```python
from build123d import *

# Parameters (mm, degrees)
CYLINDER893_R           = 1.6
CYLINDER893_DEPTH       = 10
CYLINDER893_PITCH_ANGLE = 90
CYLINDER894_R           = 1.6
CYLINDER894_DEPTH       = 10
CYLINDER894_PITCH_ANGLE = 90
CYLINDER896_R           = 3.1
CYLINDER896_DEPTH       = 2.5
CYLINDER896_PITCH_ANGLE = 90
CYLINDER895_R           = 3.1
CYLINDER895_DEPTH       = 2.5
CYLINDER895_PITCH_ANGLE = 90
BOX550_W                = 41
BOX550_H                = 41
BOX550_DEPTH            = 21
CYLINDER891_R           = 6
CYLINDER891_DEPTH       = 11
CYLINDER891_ROLL_ANGLE  = 90
CYLINDER945_R           = 7
CYLINDER945_DEPTH       = 5
CYLINDER945_ROLL_ANGLE  = 90
BOX559_W                = 10
BOX559_H                = 10
BOX559_DEPTH            = 17
CYLINDER693_R           = 1.2
CYLINDER693_DEPTH       = 10
CYLINDER693_ROLL_ANGLE  = 90
CYLINDER692_R           = 1.2
CYLINDER692_DEPTH       = 10
CYLINDER692_ROLL_ANGLE  = 90
CYLINDER697_R           = 1.25
CYLINDER697_DEPTH       = 15
CYLINDER697_PITCH_ANGLE = 90
CYLINDER695_R           = 1.25
CYLINDER695_DEPTH       = 11
CYLINDER695_PITCH_ANGLE = 90
CYLINDER696_R           = 1.25
CYLINDER696_DEPTH       = 15
CYLINDER696_PITCH_ANGLE = 90
CYLINDER694_R           = 1.25
CYLINDER694_DEPTH       = 11
CYLINDER694_PITCH_ANGLE = 90
BOX472_W                = 16
BOX472_H                = 60
BOX472_DEPTH            = 17
FILLET333_R             = 3
BOX473_W                = 10
BOX473_H                = 63
BOX473_DEPTH            = 25.5
FILLET332_R             = 3


with BuildPart() as cylinder1049:
    # Cylinder893 → Cylinder893 (new body)
    with BuildSketch(Plane.XY):
        Circle(CYLINDER893_R)
    extrude(amount=CYLINDER893_DEPTH)


with BuildPart() as cylinder1049_1:
    # Cylinder893 pitch: moved
    add(cylinder1049.part.rotate(Axis((0, 0, 0), (0, 1, 0)), CYLINDER893_PITCH_ANGLE))


with BuildPart() as cylinder1049_2:
    # Cylinder893 placement: moved
    add(cylinder1049_1.part.moved(Location((13.5, 83, -11))))


with BuildPart() as cylinder1050:
    # Cylinder894 → Cylinder894 (new body)
    with BuildSketch(Plane.XY):
        Circle(CYLINDER894_R)
    extrude(amount=CYLINDER894_DEPTH)


with BuildPart() as cylinder1050_1:
    # Cylinder894 pitch: moved
    add(cylinder1050.part.rotate(Axis((0, 0, 0), (0, 1, 0)), CYLINDER894_PITCH_ANGLE))


with BuildPart() as cylinder1050_2:
    # Cylinder894 placement: moved
    add(cylinder1050_1.part.moved(Location((13.5, 91, -11))))


with BuildPart() as cylinder1052:
    # Cylinder896 → Cylinder896 (new body)
    with BuildSketch(Plane.XY):
        Circle(CYLINDER896_R)
    extrude(amount=CYLINDER896_DEPTH)


with BuildPart() as cylinder1052_1:
    # Cylinder896 pitch: moved
    add(cylinder1052.part.rotate(Axis((0, 0, 0), (0, 1, 0)), CYLINDER896_PITCH_ANGLE))


with BuildPart() as cylinder1052_2:
    # Cylinder896 placement: moved
    add(cylinder1052_1.part.moved(Location((13.5, 83, -11))))


with BuildPart() as fusion593:
    # Cylinder895 → Cylinder895 (new body)
    with BuildSketch(Plane.XY):
        Circle(CYLINDER895_R)
    extrude(amount=CYLINDER895_DEPTH)


with BuildPart() as fusion593_1:
    # Cylinder895 pitch: moved
    add(fusion593.part.rotate(Axis((0, 0, 0), (0, 1, 0)), CYLINDER895_PITCH_ANGLE))


with BuildPart() as fusion593_2:
    # Cylinder895 placement: moved
    add(fusion593_1.part.moved(Location((13.5, 91, -11))))

    # Fusion593: union Cylinder1049, Cylinder1050, Cylinder1052
    add(cylinder1049_2.part)
    add(cylinder1050_2.part)
    add(cylinder1052_2.part)


with BuildPart() as cube741:
    # Box550 → Box550 (new body)
    with BuildSketch(Plane(origin=(19.5, 64.5, -21.5), x_dir=(1, 0, 0), z_dir=(0, 0, 1))):
        with Locations((20.5, 20.5)):
            Rectangle(BOX550_W, BOX550_H)
    extrude(amount=BOX550_DEPTH)


with BuildPart() as cylinder1048:
    # Cylinder891 → Cylinder891 (new body)
    with BuildSketch(Plane.XY):
        Circle(CYLINDER891_R)
    extrude(amount=CYLINDER891_DEPTH)


with BuildPart() as cylinder1048_1:
    # Cylinder891 roll: moved
    add(cylinder1048.part.rotate(Axis((0, 0, 0), (1, 0, 0)), CYLINDER891_ROLL_ANGLE))


with BuildPart() as cylinder1048_2:
    # Cylinder891 placement: moved
    add(cylinder1048_1.part.moved(Location((37, 64.5, -11))))


with BuildPart() as cylinder1090:
    # Cylinder945 → Cylinder945 (new body)
    with BuildSketch(Plane.XY):
        Circle(CYLINDER945_R)
    extrude(amount=CYLINDER945_DEPTH)


with BuildPart() as cylinder1090_1:
    # Cylinder945 roll: moved
    add(cylinder1090.part.rotate(Axis((0, 0, 0), (1, 0, 0)), CYLINDER945_ROLL_ANGLE))


with BuildPart() as cylinder1090_2:
    # Cylinder945 placement: moved
    add(cylinder1090_1.part.moved(Location((37, 64.5, -11))))


with BuildPart() as fusion598:
    # Box559 → Box559 (new body)
    with BuildSketch(Plane(origin=(37, 55, -19.5), x_dir=(1, 0, 0), z_dir=(0, 0, 1))):
        with Locations((5, 5)):
            Rectangle(BOX559_W, BOX559_H)
    extrude(amount=BOX559_DEPTH)

    # Fusion598: union Cube741, Cylinder1048, Cylinder1090
    add(cube741.part)
    add(cylinder1048_2.part)
    add(cylinder1090_2.part)


with BuildPart() as cylinder943:
    # Cylinder693 → Cylinder693 (new body)
    with BuildSketch(Plane.XY):
        Circle(CYLINDER693_R)
    extrude(amount=CYLINDER693_DEPTH)


with BuildPart() as cylinder943_1:
    # Cylinder693 roll: moved
    add(cylinder943.part.rotate(Axis((0, 0, 0), (1, 0, 0)), CYLINDER693_ROLL_ANGLE))


with BuildPart() as cylinder943_2:
    # Cylinder693 placement: moved
    add(cylinder943_1.part.moved(Location((3, 10, 10))))


with BuildPart() as fusion462:
    # Cylinder692 → Cylinder692 (new body)
    with BuildSketch(Plane.XY):
        Circle(CYLINDER692_R)
    extrude(amount=CYLINDER692_DEPTH)


with BuildPart() as fusion462_1:
    # Cylinder692 roll: moved
    add(fusion462.part.rotate(Axis((0, 0, 0), (1, 0, 0)), CYLINDER692_ROLL_ANGLE))


with BuildPart() as fusion462_2:
    # Cylinder692 placement: moved
    add(fusion462_1.part.moved(Location((3, 60, 10))))

    # Fusion462: union Cylinder943
    add(cylinder943_2.part)


with BuildPart() as fusion462_3:
    # Fusion462 placement: moved
    add(fusion462_2.part.moved(Location((0, 0, 2))))


with BuildPart() as cylinder976:
    # Cylinder697 → Cylinder697 (new body)
    with BuildSketch(Plane.XY):
        Circle(CYLINDER697_R)
    extrude(amount=CYLINDER697_DEPTH)


with BuildPart() as cylinder976_1:
    # Cylinder697 pitch: moved
    add(cylinder976.part.rotate(Axis((0, 0, 0), (0, 1, 0)), CYLINDER697_PITCH_ANGLE))


with BuildPart() as cylinder976_2:
    # Cylinder697 placement: moved
    add(cylinder976_1.part.moved(Location((-2, 23, 15))))


with BuildPart() as cylinder974:
    # Cylinder695 → Cylinder695 (new body)
    with BuildSketch(Plane.XY):
        Circle(CYLINDER695_R)
    extrude(amount=CYLINDER695_DEPTH)


with BuildPart() as cylinder974_1:
    # Cylinder695 pitch: moved
    add(cylinder974.part.rotate(Axis((0, 0, 0), (0, 1, 0)), CYLINDER695_PITCH_ANGLE))


with BuildPart() as cylinder974_2:
    # Cylinder695 placement: moved
    add(cylinder974_1.part.moved(Location((-2, 13.5, -1))))


with BuildPart() as cylinder975:
    # Cylinder696 → Cylinder696 (new body)
    with BuildSketch(Plane.XY):
        Circle(CYLINDER696_R)
    extrude(amount=CYLINDER696_DEPTH)


with BuildPart() as cylinder975_1:
    # Cylinder696 pitch: moved
    add(cylinder975.part.rotate(Axis((0, 0, 0), (0, 1, 0)), CYLINDER696_PITCH_ANGLE))


with BuildPart() as cylinder975_2:
    # Cylinder696 placement: moved
    add(cylinder975_1.part.moved(Location((-2, 57, 15))))


with BuildPart() as fusion463:
    # Cylinder694 → Cylinder694 (new body)
    with BuildSketch(Plane.XY):
        Circle(CYLINDER694_R)
    extrude(amount=CYLINDER694_DEPTH)


with BuildPart() as fusion463_1:
    # Cylinder694 pitch: moved
    add(fusion463.part.rotate(Axis((0, 0, 0), (0, 1, 0)), CYLINDER694_PITCH_ANGLE))


with BuildPart() as fusion463_2:
    # Cylinder694 placement: moved
    add(fusion463_1.part.moved(Location((-2, 66.5, -1))))

    # Fusion460: union Cylinder976, Cylinder974, Cylinder975
    add(cylinder976_2.part)
    add(cylinder974_2.part)
    add(cylinder975_2.part)


with BuildPart() as fusion463_3:
    # Fusion460 placement: moved
    add(fusion463_2.part.moved(Location((-10, -10, 1))))

    # Fusion463: union Fusion462
    add(fusion462_3.part)


with BuildPart() as fusion463_4:
    # Fusion463 placement: moved
    add(fusion463_3.part.moved(Location((25.5, 55, -23))))


with BuildPart() as fillet333:
    # Box472 → Box472 (new body)
    with BuildSketch(Plane(origin=(-2, 0, 1.5), x_dir=(1, 0, 0), z_dir=(0, 0, 1))):
        with Locations((8, 30)):
            Rectangle(BOX472_W, BOX472_H)
    extrude(amount=BOX472_DEPTH)

    # Fillet333
    fillet333_edges = [fillet333.edges().sort_by_distance(p)[0] for p in [
        (6, 0, 1.5),
        (6, 0, 18.5),
        (6, 60, 1.5),
        (6, 60, 18.5),
    ]]
    fillet(fillet333_edges, radius=FILLET333_R)


with BuildPart() as fillet333_1:
    # Fillet333 placement: moved
    add(fillet333.part.moved(Location((25.5, 55, -21))))


with BuildPart() as cross_member_front:
    # Box473 → Box473 (new body)
    with BuildSketch(Plane(origin=(-12, 0, -5), x_dir=(1, 0, 0), z_dir=(0, 0, 1))):
        with Locations((5, 31.5)):
            Rectangle(BOX473_W, BOX473_H)
    extrude(amount=BOX473_DEPTH)

    # Fillet332
    fillet332_edges = [cross_member_front.edges().sort_by_distance(p)[0] for p in [
        (-7, 0, -5),
        (-7, 0, 20.5),
        (-7, 63, -5),
        (-7, 63, 20.5),
    ]]
    fillet(fillet332_edges, radius=FILLET332_R)


with BuildPart() as cross_member_front_1:
    # Fillet332 placement: moved
    add(cross_member_front.part.moved(Location((25.5, 53.5, -21.5))))

    # Fusion464: union Fillet333
    add(fillet333_1.part)

    # Cut581: cut Fusion463
    add(fusion463_4.part, mode=Mode.SUBTRACT)

    # Cut696: cut Fusion598
    add(fusion598.part, mode=Mode.SUBTRACT)

    # Cut697: cut Fusion593
    add(fusion593_2.part, mode=Mode.SUBTRACT)


solid = cross_member_front_1.part
```
Geometry check sheet. Reference: the model listing, model coordinates, mm. A direction names the side the tool comes from. Coordinates: 2 decimals unless noted, no trailing zeros. Order: outer loops, then holes, each group sorted by start corner. A loop starts at its lowest first (then second) coordinate and runs counter-clockwise, first axis right, second up. Notation, with made-up numbers: M -28.75,32 L 28.25,32 A28 ccw 28.25,71 Z; hole C 4,-12.75 d3. An arc over 180 degrees is marked long. Answer as a JSON object with one key per item and string values.
Q1. Release check for a two-part mould opening along Y. For faces 4 (the cylindrical face through (17.73, 83.07, -9.4)), 5 (the flat face through (39.5, 110, -11)), 6 (the cylindrical face through (31.61, 114.14, -3.4)) record: released by +Y, released by -Y, zero draft, split by the parting line, or undercut.
Results are:
{"face 4": "undercut", "face 5": "zero draft", "face 6": "released by +Y"}
Q2. Cross-section at B-B on x = 28.5. Record the cut outline in (y, z).
Results are:
{"outline": "M 55,-16.5 A3 ccw 58,-19.5 L 64.5,-19.5 L 64.5,-12.2 L 55,-12.2 Z; M 55,-9.8 L 64.5,-9.8 L 64.5,-2.5 L 58,-2.5 A3 ccw 55,-5.5 Z; M 105.5,-19.5 L 112,-19.5 A3 ccw 115,-16.5 L 115,-12.2 L 105.5,-12.2 Z; M 105.5,-9.8 L 115,-9.8 L 115,-5.5 A3 ccw 112,-2.5 L 105.5,-2.5 Z"}
Q3. Cross-section at D-D on z = -11. Give the number of separate pieces and of enclosed holes in the cut face, and give its area (3 significant figures).
Results are:
{"separate pieces": "5", "enclosed holes": "0", "area": "585 mm²"}
Q4. Scan lines: line 1 (Y direction, x = 15.05, z = -11); line 2 (Y direction, x = 17.7, z = -11); line 3 (Y direction, x = 27.25, z = -6). Record each from-to range of solid material in increasing order.
Results are:
{"line 1": "y = 53.5 to 79.9, 86.1 to 87.9, 94.1 to 116.5", "line 2": "y = 53.5 to 81.4, 84.6 to 89.4, 92.6 to 116.5", "line 3": "y = 55 to 64.5, 105.5 to 115"}
Q5. Cross-section at A-A on y = 91. Record the cut outline in (x, z), and give its area (3 significant figures).
Results are:
{"outline": "M 13.5,-26.5 L 23.5,-26.5 L 23.5,-21.5 L 19.5,-21.5 L 19.5,-12.6 L 16,-12.6 L 16,-14.1 L 13.5,-14.1 Z; M 13.5,-7.9 L 16,-7.9 L 16,-9.4 L 19.5,-9.4 L 19.5,-1 L 13.5,-1 Z", "area": "146 mm²"}
Q6. Depth check by flat-ended pin: pin 1 Ø1.5 at (x, z) = (33, -6.5) entering from +Y; pin 2 Ø2.5 at (y, z) = (91, -11) entering from +X; pin 3 Ø5 at (y, z) = (91, -11) entering from +X; pin 4 Ø10 at (x, z) = (33.5, -13.5) entering from -Y. Enter the tip coordinate at first touch or a pass-through.
Results are:
{"pin 1": "stops at y = 115", "pin 2": "passes through", "pin 3": "stops at x = 19.5", "pin 4": "stops at y = 55"}
Q7. Tool access check on faces 1 (the flat face through (16, 89.7, -12.3)), 2 (the flat face through (37, 60, -3)), 3 (the flat face through (21, 85, -21.5)). Record the directions out of +Z, -Z, +X, -X, +Y, -Y that give a thin tool (end or side, any length) a straight path to the whole face; none if there is none.
Results are:
{"face 1": "-X", "face 2": "+Z, -Z, +X, -Y", "face 3": "+Z, +X"}
Q8. Cross-section at C-C on y = 70.5. Record the cut outline in (x, z), and give its area (3 significant figures).
Results are:
{"outline": "M 13.5,-26.5 L 23.5,-26.5 L 23.5,-21.5 L 19.5,-21.5 L 19.5,-1 L 13.5,-1 Z", "area": "173 mm²"}
